Can you work these out from the drawing? Everything is in mm from the part's minimum corner. A direction names the side the tool comes from. Give positions to 0.01 mm unless a question says otherwise; leave off trailing zeros. Loops run counter-clockwise (first coordinate to the right, second up) from the corner with the lowest first, then second, coordinate; pieces in that order, holes last. Notation, with made-up numbers: M 71.5,-24.75 L 93.5,-24.75 A30 ccw 93.5,13.25 Z; hole C 81.5,46.5 d6. An arc over 180 degrees is marked long. Use CSV: the item, a comma, the result in double quotes.
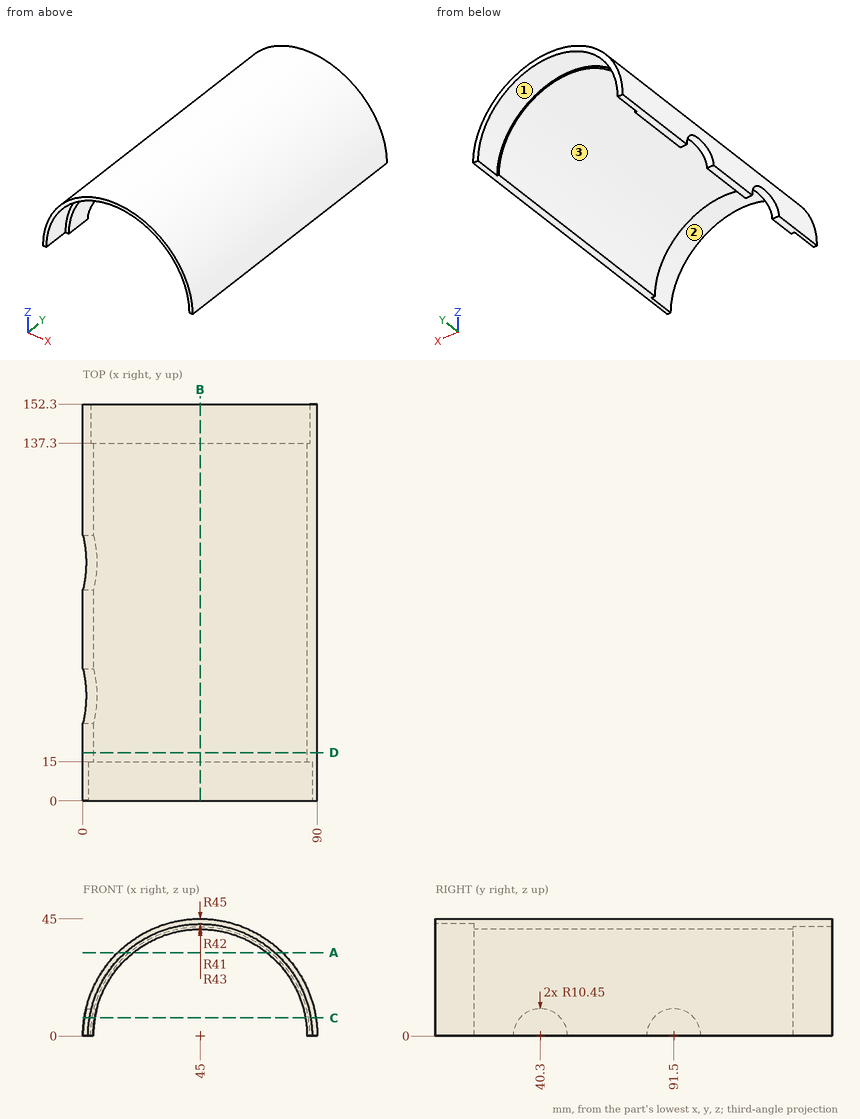
Q1. I want a section at C-C, the plane z = 7. Please give me the cut outline in (x, y).
Model answer:
outline,"M 0.55,0 L 2.57,0 L 2.57,15 L 4.6,15 L 4.6,32.54 L 0.55,32.54 Z; M 0.55,48.06 L 4.6,48.06 L 4.6,83.74 L 0.55,83.74 Z; M 0.55,99.26 L 4.6,99.26 L 4.6,137.3 L 3.59,137.3 L 3.59,152.3 L 0.55,152.3 Z; M 85.4,15 L 87.43,15 L 87.43,0 L 89.45,0 L 89.45,152.3 L 86.41,152.3 L 86.41,137.3 L 85.4,137.3 Z"
Q2. I'm going to push flat-ended pins straight in: P1, Ø2, axis at y = 71, z = 23, coming from the -X side; P2, Ø10, axis at x = 23, y = 109, coming from the -Z side; P3, Ø5, axis at y = 105.5, z = 29.5, coming from the +X side. Where does each tip first touch, or does it pass through?
Model answer:
P1,"x = 5.74"
P2,"z = 30.85"
P3,"x = 81"
Q3. I want a section at B-B, the plane x = 45. Please give me the cut outline in (y, z), then the cut area to 3 significant figures.
Model answer:
outline,"M 0,43 L 15,43 L 15,41 L 137.3,41 L 137.3,42 L 152.3,42 L 152.3,45 L 0,45 Z"
area,"564 mm2"
Q4. Please list where these lines run through material, in increasing order: L1, parallel to X at y = 29, z = 9; L2, parallel to X at y = 90, z = 17; L3, parallel to Y at x = 86, z = 10.5. Write a range as from..to.
Model answer:
L1,"0.91..5, 85..89.09"
L2,"3.33..7.69, 82.31..86.67"
L3,"15..152.3"
Q5. I want a section at A-A, the plane z = 32. Please give me the cut outline in (x, y), then the cut area to 3 significant figures.
Model answer:
outline,"M 13.36,0 L 16.28,0 L 16.28,15 L 19.37,15 L 19.37,137.3 L 17.8,137.3 L 17.8,152.3 L 13.36,152.3 Z; M 70.63,15 L 73.72,15 L 73.72,0 L 76.64,0 L 76.64,152.3 L 72.2,152.3 L 72.2,137.3 L 70.63,137.3 Z"
area,"1,690 mm2"
Q6. For the marked faces 1, 2 and 3, which set-ups out of +Z, -Z, +X, -X, +Y, -Y let a thin tool reach every point of the face, with its end or its side?
Model answer:
face 1,"-Z, +Y"
face 2,"-Z, -Y"
face 3,"-Z, +Y, -Y"
Q7. I want a section at D-D, the plane y = 18.5. Please give me the cut outline in (x, z), then the cut area to 3 significant figures.
Model answer:
outline,"M 0,0 L 4,0 A41 cw 86,0 L 90,0 A45 ccw Z"
area,"540 mm2"
